Autodesk Inventor part; units mm, degrees
ref_plane "YZ Plane" through (0, 0, 0) normal (1, 0, 0) x (0, 1, 0)
ref_plane "XZ Plane" through (0, 0, 0) normal (0, 1, 0) x (-1, 0, 0)
ref_plane "XY Plane" through (0, 0, 0) normal (0, 0, 1) x (1, 0, 0)
sketch "Эскиз1" plane through (0, 0, 0) normal (1, 0, 0) x (0, 1, 0)
  circle A0 centre (0, 0) radius 14
  dimension "d0" = 28
extrude "Выдавливание1" add sketch "Эскиз1" along normal mid plane 45
sketch "Эскиз2" plane through (22.5, 0, 0) normal (1, 0, 0) x (0, 0, -1)
  point P0 (0, 0)
  point P1 (0, 0)
hole "Отверстие1" at (22.5, 0, 0) direction (-1, 0, 0) diameter 6 depth 60
fillet "Сопряжение1" radius 0.2 2 edges at (22.5, 0, 3) (-22.5, 0, 3)
ref_plane "РабПлоскость2" through (-14.5, 2.1629, 84.9725) normal (-1, 0, 0) x (0, -0.9996762, 0.0254464)
sketch "Эскиз4" plane through (-14.5, 2.1629, 84.9725) normal (-1, 0, 0) x (0, -0.9996762, 0.0254464)
  circle A0 centre (0, -85) radius 10
  circle A1 centre (0, -85) radius 3.2
  circle A2 centre (0, -85) radius 14
  dimension "d14" = 20
extrude "Выдавливание3" cut sketch "Эскиз4" against normal blind 12 contours A2
properties part number "Вал конвейера"
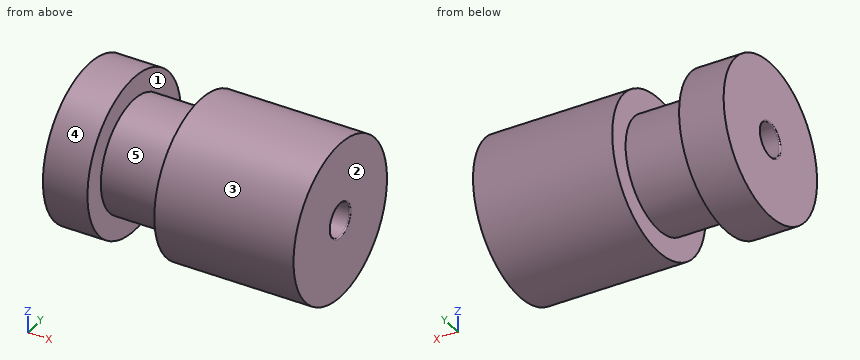
Geometry check sheet. Reference: the model listing, model coordinates, mm. Face numbers are marked on the shaded views. A direction names the side the tool comes from. Round coordinates to 2 decimals unless told otherwise and drop trailing zeros. Write each loop counter-clockwise with the first axis right and the second up, starting at its lowest first coordinate (ties: lowest second). Pieces come first, ordered by that corner, then holes. Notation, with made-up numbers: (33, -38.5) - (77, -38.5) arc R26 cw to (77, -12.5) - close; hole circle Ø5 at (71, -0.75). An arc over 180 degrees is marked (long way). One line per item, written item: value.
1. Depth check by flat-ended pin: pin 1 Ø12 at (x, y) = (1.5, 10) entering from -Z; pin 2 Ø4 at (x, z) = (-0.5, -6) entering from -Y; pin 3 Ø1.5 at (x, z) = (2.5, 3) entering from +Y. Enter the tip coordinate at first touch or a pass-through.
The answers:
pin 1: stops at z = -13.42
pin 2: stops at y = -13.42
pin 3: stops at y = 13.82
2. Cross-section at A-A on y = 0. Record the boundary of the cut face in (x, z), and give its area (3 significant figures).
The answers:
outline: (-22.5, -14) - (-14.5, -14) - (-14.5, -10) - (-2.5, -10) - (-2.5, -14) - (22.5, -14) - (22.5, -3.2) arc R0.2 ccw to (22.3, -3) - (-22.3, -3) arc R0.2 ccw to (-22.5, -3.2) - close; (-22.5, 3.2) arc R0.2 ccw to (-22.3, 3) - (22.3, 3) arc R0.2 ccw to (22.5, 3.2) - (22.5, 14) - (-2.5, 14) - (-2.5, 10) - (-14.5, 10) - (-14.5, 14) - (-22.5, 14) - close
area: 894 mm^2
3. Mould release check, pull along X, two halves, no side actions. Record for the marked faces 1, 2 and 3: released by +X, released by -X, zero draft, split by the parting line, or undercut.
The answers:
face 1: undercut
face 2: released by +X
face 3: zero draft
4. Cross-section at B-B on z = -5. Record the boundary of the cut face in (x, y), and give its area (3 significant figures).
The answers:
outline: (-22.5, -13.08) - (-14.5, -13.08) - (-14.5, -8.66) - (-2.5, -8.66) - (-2.5, -13.08) - (22.5, -13.08) - (22.5, 13.08) - (-2.5, 13.08) - (-2.5, 8.66) - (-14.5, 8.66) - (-14.5, 13.08) - (-22.5, 13.08) - close
area: 1,070 mm^2
5. Cross-section at D-D on x = -16. Record the boundary of the cut face in (y, z).
The answers:
outline: circle Ø28 at (0, 0); hole circle Ø6 at (0, 0)
6. Cross-section at C-C on y = 4.75. Record the boundary of the cut face in (x, z).
The answers:
outline: (-22.5, -13.17) - (-14.5, -13.17) - (-14.5, -8.8) - (-2.5, -8.8) - (-2.5, -13.17) - (22.5, -13.17) - (22.5, 13.17) - (-2.5, 13.17) - (-2.5, 8.8) - (-14.5, 8.8) - (-14.5, 13.17) - (-22.5, 13.17) - close
7. Scan lines: L1, parallel to X at y = -8.75, z = -6.25; L2, parallel to Z at x = -13, y = 0; L3, parallel to Z at x = -2, y = 0. Record each from-to range of solid material in increasing order.
The answers:
L1: x = -22.5 to -14.5, -2.5 to 22.5
L2: z = -10 to -3, 3 to 10
L3: z = -14 to -3, 3 to 14
8. Set-up check for the marked faces 4 and 5: record each of +Z, -Z, +X, -X, +Y, -Y from which the full face is reachable in a straight line by a thin tool's end or side.
The answers:
face 4: +X, -X
face 5: none
